Part model, mm, in its own coordinate system. Round coordinates to 2 decimals unless told otherwise and drop trailing zeros. Answer as a JSON object with one key per item and string values. Group by question number.
from build123d import *

# Parameters (mm, degrees)
SKETCH1_R           = 2.1
BOSS_EXTRUDE1_DEPTH = 500
FILLET1_R           = 0.5


with BuildPart() as part:
    # Sketch1 → Boss-Extrude1 (new body)
    with BuildSketch(Plane.XY):
        Polygon((2.839339828, 13.9), (5.5, 16.560660172), (5.5, 18.2), (3.125, 18.2), (3.125, 18.545), (4.58, 20), (10, 20), (10, 14.58), (8.545, 13.125), (8.2, 13.125), (8.2, 15.5), (6.560660172, 15.5), (3.9, 12.839339828), (3.9, 10.2), (3.7, 10), (3.9, 9.8), (3.9, 7.160660172), (6.560660172, 4.5), (8.2, 4.5), (8.2, 6.875), (8.545, 6.875), (10, 5.42), (10, -5.42), (8.545, -6.875), (8.2, -6.875), (8.2, -4.5), (6.560660172, -4.5), (3.9, -7.160660172), (3.9, -9.8), (3.7, -10), (3.9, -10.2), (3.9, -12.839339828), (6.560660172, -15.5), (8.2, -15.5), (8.2, -13.125), (8.545, -13.125), (10, -14.58), (10, -20), (4.58, -20), (3.125, -18.545), (3.125, -18.2), (5.5, -18.2), (5.5, -16.560660172), (2.839339828, -13.9), (0.2, -13.9), (0, -13.7), (-0.2, -13.9), (-2.839339828, -13.9), (-5.5, -16.560660172), (-5.5, -18.2), (-3.125, -18.2), (-3.125, -18.545), (-4.58, -20), (-10, -20), (-10, -14.58), (-8.545, -13.125), (-8.2, -13.125), (-8.2, -15.5), (-6.560660172, -15.5), (-3.9, -12.839339828), (-3.9, -10.2), (-3.7, -10), (-3.9, -9.8), (-3.9, -7.160660172), (-6.560660172, -4.5), (-8.2, -4.5), (-8.2, -6.875), (-8.545, -6.875), (-10, -5.42), (-10, 5.42), (-8.545, 6.875), (-8.2, 6.875), (-8.2, 4.5), (-6.560660172, 4.5), (-3.9, 7.160660172), (-3.9, 9.8), (-3.7, 10), (-3.9, 10.2), (-3.9, 12.839339828), (-6.560660172, 15.5), (-8.2, 15.5), (-8.2, 13.125), (-8.545, 13.125), (-10, 14.58), (-10, 20), (-4.58, 20), (-3.125, 18.545), (-3.125, 18.2), (-5.5, 18.2), (-5.5, 16.560660172), (-2.839339828, 13.9), (-0.2, 13.9), (0, 13.7), (0.2, 13.9), align=None)
        with Locations((0, 10)):
            Circle(SKETCH1_R, mode=Mode.SUBTRACT)
        with Locations((0, -10)):
            Circle(SKETCH1_R, mode=Mode.SUBTRACT)
        Polygon((8.2, -3), (8.2, 3), (5.939339828, 3), (2.839339828, 6.1), (0.2, 6.1), (0, 6.3), (-0.2, 6.1), (-2.839339828, 6.1), (-5.939339828, 3), (-8.2, 3), (-8.2, -3), (-5.939339828, -3), (-2.839339828, -6.1), (-0.2, -6.1), (0, -6.3), (0.2, -6.1), (2.839339828, -6.1), (5.939339828, -3), align=None, mode=Mode.SUBTRACT)
    extrude(amount=BOSS_EXTRUDE1_DEPTH)

    # Fillet1
    fillet1_edges = [part.edges().sort_by_distance(p)[0] for p in [
        (10, -20, 250),
        (-10, -20, 250),
        (-10, 20, 250),
        (10, 20, 250),
    ]]
    fillet(fillet1_edges, radius=FILLET1_R)


solid = part.part
Item 1: Band-saw the part on A-A, the plane z = 86. Count the separate pieces of the cut face and the enclosed holes in it, plus the area to 3 significant figures.
Item 2: Drop flat-ended pins along their axis: pin 1 Ø6 at (y, z) = (10, 189) entering from +X; pin 2 Ø8 at (x, y) = (2, -5) entering from -Z; pin 3 Ø2 at (y, z) = (10.5, 134) entering from -X; pin 4 Ø2 at (y, z) = (-12, 256.5) entering from -X. Give the stop position or say it passes through.
Item 3: Drill centre lines: line 1 (Y direction, x = 0, z = 130); line 2 (Y direction, x = -0.25, z = 31); line 3 (Y direction, x = -4.25, z = 36). Where is each one in solid material? Low to high.
Entries:
{
 "1": {"separate pieces": "1", "enclosed holes": "3", "area": "297 mm²"},
 "2": {"pin 1": "x = 4.06", "pin 2": "z = 0", "pin 3": "x = -3.9", "pin 4": "x = -4.06"},
 "3": {"line 1": "-13.7 to -12.1, -7.9 to -6.3, 6.3 to 7.9, 12.1 to 13.7", "line 2": "-13.9 to -12.09, -7.91 to -6.1, 6.1 to 7.91, 12.09 to 13.9", "line 3": "-19.67 to -18.2, -15.31 to -13.19, -6.81 to -4.69, 4.69 to 6.81, 13.19 to 15.31, 18.2 to 19.67"}
}
